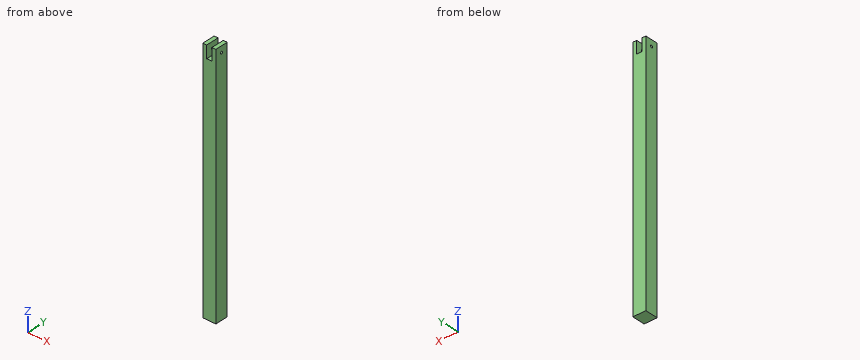
from build123d import *

# Parameters (mm, degrees)
ESQUISSE1_W             = 90
ESQUISSE1_H             = 90
BOSS_EXTRU_1_DEPTH      = 1700
ESQUISSE2_W             = 36
ESQUISSE2_H             = 85
ENL_V_MAT_EXTRU_1_DEPTH = 1705.758047349
ESQUISSE3_R             = 8
ENL_V_MAT_EXTRU_2_DEPTH = 1705.758047349


with BuildPart() as part:
    # Esquisse1 → Boss.-Extru.1 (new body)
    with BuildSketch(Plane.XY):
        with Locations((45, 45)):
            Rectangle(ESQUISSE1_W, ESQUISSE1_H)
    extrude(amount=BOSS_EXTRU_1_DEPTH)

    # Esquisse2 → Enlèv. mat.-Extru.1 (cut, through all)
    with BuildSketch(Plane.XZ):
        with Locations((45, 1657.5)):
            Rectangle(ESQUISSE2_W, ESQUISSE2_H)
    extrude(amount=-ENL_V_MAT_EXTRU_1_DEPTH, mode=Mode.SUBTRACT)

    # Esquisse3 → Enlèv. mat.-Extru.2 (cut, through all)
    with BuildSketch(Plane(origin=(90, 0, 0), x_dir=(0, 0, -1), z_dir=(1, 0, 0))):
        with Locations((-1657.5, 45)):
            Circle(ESQUISSE3_R)
    extrude(amount=-ENL_V_MAT_EXTRU_2_DEPTH, mode=Mode.SUBTRACT)


solid = part.part
Build history of the part. All positions in model axes, mm. Give positions to 0.01 mm unless a question says otherwise; leave off trailing zeros. Order: outer loops, then holes, each group sorted by start corner. A loop starts at its lowest first (then second) coordinate and runs counter-clockwise, first axis right, second up. Notation, with made-up numbers: M 79,-1 L 102,-1 A19 ccw 102,25 Z; hole C 57.25,35.25 d3. An arc over 180 degrees is marked long. Put each result on its own line as item: value.
Item 1: Probe line 1 (Y direction, x = 83, z = 1657); line 2 (Z direction, x = 28, y = 65). List the from-to ranges inside material, lowest first. Write a range as [from, to].
From the geometry:
line 1: y = [0, 37.02], [52.98, 90]
line 2: z = [0, 1615]
Item 2: Slice it at A-A, the plane y = 19. Write the cut outline in (x, z).
From the geometry:
outline: M 0,0 L 90,0 L 90,1700 L 63,1700 L 63,1615 L 27,1615 L 27,1700 L 0,1700 Z
Item 3: Flat gauge pins, fed straight in: pin 1 Ø18 at (x, y) = (41.5, 47) entering from +Z; pin 2 Ø9.5 at (y, z) = (45, 1657.5) entering from +X. Where does each tip first touch, or does it go through?
From the geometry:
pin 1: stops at z = 1615
pin 2: passes through
